Part model, mm, in its own coordinate system. A direction names the side the tool comes from. Round coordinates to 2 decimals unless told otherwise and drop trailing zeros. Use CSV: the item, a comma, the result in double quotes. Start each with the question number.
(1) Which spindle directions (+Z, -Z, +X, -X, +Y, -Y) get a long thin tool onto all of the face, cutting with end or side? Do faces 1 (the cylindrical face through (350.533, 183.987, -1.802)), 2 (the flat face through (354, 566, 39.5)). Say none if no direction does.
(2) Drop flat-ended pins along their axis: pin 1 (6 mm diameter, centred on x = 345.5, y = 197.5, fed in from +Z); pin 2 (5 mm diameter, centred on x = 354, y = 291, fed in from +Z); pin 3 (2 mm diameter, centred on x = 347, z = 0.5, fed in from +Y). Give the stop position or say it passes through.
(3) Probe line 1 (Y direction, x = 335.5, z = 23); line 2 (Y direction, x = 363.5, z = 15); line 3 (Y direction, x = 327.5, z = 2.5). List the from-to ranges inside material, lowest first. Write a range as [from, to].
```python
from build123d import *

# Parameters (mm, degrees)
CHAMFER1_SIZE       = 5
CHAMFER2_SIZE       = 2
SKETCH2_W           = 51
SKETCH2_H           = 79
BOSS_EXTRUDE1_DEPTH = 71
FILLET1_R           = 2


with BuildPart() as part:
    # Sketch1 → Revolve2 (revolve)
    with BuildSketch(Plane.XY):
        Polygon((387.82109188, 517.961255794), (388.108543141, 529.957812458), (353.118586206, 530.796211969), (340.38333201, -0.699799139), (346.381610341, -0.843524769), (355.116501156, 363.700406109), (374.860833998, 363.227309242), (375.076422443, 372.22472674), (383.823911677, 372.015126862), (384.638356916, 406.005370741), (365.643808866, 406.460501904), (365.907305855, 417.457345512), (370.406014604, 417.349551289), (371.867225181, 478.33204766), (378.865216568, 478.164367758), (379.344302003, 498.158628863), (384.342867279, 498.038857504), (384.479406628, 503.737221919), (380.980410934, 503.82106187), (381.186417671, 512.418594146), (384.685413365, 512.334754195), (384.821952714, 518.03311861), align=None)
    revolve(axis=Axis((340.38333201, -0.699799139, 0), (0.023954271746676543, 0.9997130552639024, 0)))

    # Chamfer1
    # the kernel refuses this chamfer: 5 mm, written as the material it takes off along each edge
    with BuildSketch(Plane(origin=(350.411753499, 417.828636724, 0), x_dir=(0.9997130552639024, -0.02395427174667721, 0), z_dir=(0, 0, 1))) as chamfer1_piece_1_section:
        Polygon((20 - CHAMFER1_SIZE, 0), (20, CHAMFER1_SIZE), (20, 0), align=None)
    chamfer1_piece_1 = revolve(axis=Axis((350.411753499, 417.828636724, 0), (0.023954271746676543, 0.9997130552639024, 0)), mode=Mode.PRIVATE)
    chamfer1_piece_1 = chamfer1_piece_1 - Plane(origin=(350.477356387, 420.56652265, 0), x_dir=(0.9997130552639024, -0.023954271746676543, 0), z_dir=(0.023954271746676543, 0.9997130552639024, 0)) * Cylinder(15.5, 80, mode=Mode.PRIVATE)
    add(chamfer1_piece_1, mode=Mode.SUBTRACT)

    # Chamfer2
    chamfer2_edges = [part.edges().sort_by_distance(p)[0] for p in [
        (324.880711583, 479.457898432, 0),
        (323.375611652, 364.460954237, 0),
    ]]
    chamfer(chamfer2_edges, length=CHAMFER2_SIZE)

    # Sketch2 → Boss-Extrude1 (add)
    with BuildSketch(Plane(origin=(12.913810212, 538.947908709, 0), x_dir=(0.9997130552639024, -0.023954271746676654, 0), z_dir=(0.023954271746676657, 0.9997130552639025, 0))):
        with Locations((340.302423983, 0)):
            Rectangle(SKETCH2_W, SKETCH2_H)
    extrude(amount=BOSS_EXTRUDE1_DEPTH)

    # Fillet1
    fillet1_edges = [part.edges().sort_by_distance(p)[0] for p in [
        (328.476279944, 566.89685936, -39.5),
        (328.476279944, 566.89685936, 39.5),
        (379.461645763, 565.675191501, 39.5),
        (379.461645763, 565.675191501, -39.5),
    ]]
    fillet(fillet1_edges, radius=FILLET1_R)


solid = part.part
```
Answers:
1,face 1,"none"
1,face 2,"+Z, +X, -X, +Y, -Y"
2,pin 1,"stops at z = 6"
2,pin 2,"stops at z = 4.36"
2,pin 3,"stops at y = 601.99"
3,line 1,"y = [373.17, 407.18], [499.21, 504.91], [513.51, 602.24]"
3,line 2,"y = [363.5, 406.51], [422.35, 601.57]"
3,line 3,"y = [364.36, 407.37], [479.4, 531.41]"
